Check sheet for the modelled part. Datum: model origin and axes. Units: mm. Face numbers are marked on the shaded views. A direction names the side the tool comes from. Round coordinates to 2 decimals unless told otherwise and drop trailing zeros. Loops run counter-clockwise (first coordinate to the right, second up) from the corner with the lowest first, then second, coordinate; pieces in that order, holes last. Notation, with made-up numbers: M 74.25,37 L 126.25,37 A21 ccw 126.25,53 Z; hole C 27,17 d7. An arc over 180 degrees is marked long. One line per question, with ' | ' between items. Start each with the question number.
(1) Section check B-B (z = 12). Record the boundary of the cut face in (x, y).
(2) Draft check along X on the marked faces 1, 2 and 3. Enter one of: +X half, -X half, draft (parallel to the pull), parting line (faces both ways), or undercut.
(3) Thickness scan on probe 1 along Y at (x, z) = (0, 1); probe 2 along Z at (x, y) = (-36, -33.75); probe 3 along Y at (x, z) = (0, 8.75). Record the ranges inside material, lowest first. Write a range as [from, to].
(4) Tool access check on the marked faces 4, 5 and 6. Record the directions out of +Z, -Z, +X, -X, +Y, -Y that give a thin tool (end or side, any length) a straight path to the whole face; none if there is none.
(5) Section check D-D (y = 0). Record the boundary of the cut face in (x, z).
(6) Section check A-A (z = 7.5). Record the boundary of the cut face in (x, y).
(7) Go/stop test with flat-tipped pins: P1, Ø1, axis at y = 3.5, z = 12.5, coming from the -X side; P2, Ø4.5, axis at x = -37, z = 4, coming from the +Y side; P3, Ø6, axis at y = 19.5, z = 6.5, coming from the +X side; P4, Ø5, axis at x = 36, z = 7.5, coming from the -Y side. Record where each tip stops, or that it passes through.
(8) Section check C-C (x = 0). Record the boundary of the cut face in (y, z).
```python
from build123d import *

# Parameters (mm, degrees)
SKETCH_1_R          = 23.5
EXTRUDE_1_DEPTH     = 15
SKETCH_1_3_R        = 23.5
SKETCH_1_3_R_2      = 18.5
EXTRUDE_2_DEPTH     = 3
SKETCH_2_R          = 3
CUT_EXTRUDE_1_DEPTH = 75.42781738


with BuildPart() as part:
    # Sketch 1 → Extrude 1 (new body)
    with BuildSketch(Plane.XY):
        Polygon((28.5, -30), (28.5, 18.5), (18.5, 28.5), (-18.5, 28.5), (-28.5, 18.5), (-28.5, -30), (-43.5, -30), (-43.5, -45), (43.5, -45), (43.5, -30), align=None)
        Circle(SKETCH_1_R, mode=Mode.SUBTRACT)
    extrude(amount=EXTRUDE_1_DEPTH)

    # Sketch 1_3 → Extrude 2 (add)
    with BuildSketch(Plane.XY):
        Circle(SKETCH_1_3_R)
        Circle(SKETCH_1_3_R_2, mode=Mode.SUBTRACT)
    extrude(amount=EXTRUDE_2_DEPTH)

    # Sketch 2 → Cut-Extrude 1 (cut, through all)
    with BuildSketch(Plane(origin=(0, -30, 0), x_dir=(1, 0, 0), z_dir=(0, 1, 0))):
        with Locations(Location((-36, -7.5, 0), (0, 0, 180))):
            Circle(SKETCH_2_R)
    cut_extrude_1 = extrude(amount=-CUT_EXTRUDE_1_DEPTH, mode=Mode.SUBTRACT)

    # Mirror 1: Cut-Extrude 1 across plane
    add(cut_extrude_1.mirror(Plane(origin=(0, 0, 0), x_dir=(0, 0, 1), z_dir=(1, 0, 0))), mode=Mode.SUBTRACT)


solid = part.part
```
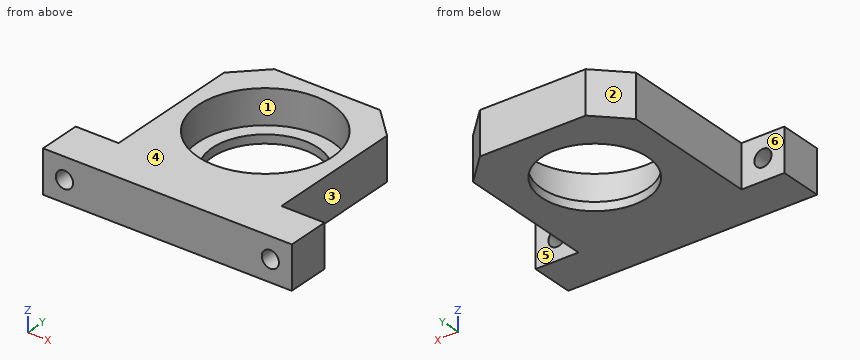
The answers:
1) outline: M -43.5,-45 L 43.5,-45 L 43.5,-30 L 28.5,-30 L 28.5,18.5 L 18.5,28.5 L -18.5,28.5 L -28.5,18.5 L -28.5,-30 L -43.5,-30 Z; hole C 0,0 d47
2) face 1: undercut | face 2: -X half | face 3: +X half
3) probe 1: [-45, -18.5], [18.5, 28.5] | probe 2: [0, 4.5], [10.5, 15] | probe 3: [-45, -23.5], [23.5, 28.5]
4) face 4: +Z, +X, -X, +Y, -Y | face 5: +Z, -Z, +X, +Y | face 6: +Z, -Z, -X, +Y
5) outline: M -28.5,0 L -18.5,0 L -18.5,3 L -23.5,3 L -23.5,15 L -28.5,15 Z; M 18.5,0 L 28.5,0 L 28.5,15 L 23.5,15 L 23.5,3 L 18.5,3 Z
6) outline: M -43.5,-45 L -39,-45 L -39,-30 L -43.5,-30 Z; M -33,-45 L 33,-45 L 33,-30 L 28.5,-30 L 28.5,18.5 L 18.5,28.5 L -18.5,28.5 L -28.5,18.5 L -28.5,-30 L -33,-30 Z; M 39,-45 L 43.5,-45 L 43.5,-30 L 39,-30 Z; hole C 0,0 d47
7) P1: x = -28.5 | P2: y = -30 | P3: x = 28.5 | P4: through
8) outline: M -45,0 L -18.5,0 L -18.5,3 L -23.5,3 L -23.5,15 L -45,15 Z; M 18.5,0 L 28.5,0 L 28.5,15 L 23.5,15 L 23.5,3 L 18.5,3 Z
